Source: CAD feature listing. Evaluate the final solid. Frame: model axes, mm. A direction names the side the tool comes from. Give positions to 0.01 mm unless a question says otherwise; leave off trailing zeros. One line per question, with ' | ' between items. Start each with the question number.
(1) Section A-A, the plane z = 0. State how many separate pieces and enclosed holes the cut face has, plus the area to 3 significant figures.
(2) Ray query, line 1 (X direction, y = 115, z = 17); line 2 (X direction, y = 102, z = 22); line 3 (Z direction, x = -19.5, y = 96). Return the intervals inside material, ascending. Write a range as [from, to].
(3) Access query for faces 1 (the cylindrical face through (-6.93, 62.64, -31.22)), 2 (the cylindrical face through (-1.384, 3.909, 40.762)). Directions: +Z, -Z, +X, -X, +Y, -Y. A direction counts if a zero-diameter tool reaches every point of the face in a straight line with its end or side. Return the directions, or none.
(4) Pin query (flat end, axial travel): pin 1 (6 mm diameter, centred on x = 15, y = 47, fed in from -Z); pin 2 (12 mm diameter, centred on x = 23, z = 27.5, fed in from -Y); pin 3 (5 mm diameter, centred on x = 6.5, y = 77, fed in from -Z); pin 4 (8 mm diameter, centred on x = -33, z = -19.05, fed in from +Y). Return the tip coordinate at first contact, or that it passes through.
Autodesk Inventor part; units mm, degrees
ref_plane "YZ Plane" through (0, 0, 0) normal (1, 0, 0) x (0, 1, 0)
ref_plane "XZ Plane" through (0, 0, 0) normal (0, 1, 0) x (-1, 0, 0)
ref_plane "XY Plane" through (0, 0, 0) normal (0, 0, 1) x (1, 0, 0)
sketch "Sketch1" plane through (0, 0, 0) normal (0, 0, 1) x (1, 0, 0)
  line L0 (0, 0) -> (0, 25.4) construction
  line L1 (30.48, 0) -> (30.48, 127)
  line L2 (0, 0) -> (30.48, 0)
  arc A0 (30.48, 0) -> (30.48, 127) centre (13.335, 63.5) ccw
  line L3 (31.98, 125.0101) -> (31.98, 1.9899)
  arc A1 (31.98, 1.9899) -> (31.98, 125.0101) centre (13.335, 63.5) ccw
  dimension "d0" = 25.4
  dimension "d1" = 30.48
  dimension "d2" = 127
  dimension "d8" = 17.145
  dimension "d9" = 1.5
revolve "Revolution1" add sketch "Sketch1" angle 360 about axis through (0, 0, 0) along (0, 1, 0)
sketch "Sketch2" plane through (0, 0, 0) normal (0, 1, 0) x (-1, 0, 0)
  circle A0 centre (0, 38.1) radius 3
  line L0 (0, 0) -> (0, 38.1) construction
  dimension "d11" = 6
  dimension "d12" = 38.1
extrude "Extrusion1" cut sketch "Sketch2" along normal blind 127
pattern_circular "Circular Pattern1" count 3 over 360 about axis through (0, 63.5, 0) along (0, 1, 0) of "Extrusion1"
properties part number "Buoy 5 HalfSphere"
Check sheet entries:
1) separate pieces: 2 | enclosed holes: 2 | area: 879 mm²
2) line 1: [-51.52, -48.92], [-27.09, -25.3], [25.3, 27.09], [48.92, 51.52] | line 2: [-62.93, -60.95], [-23.21, -21.1], [21.1, 23.21], [60.95, 62.93] | line 3: [-67.77, -65.96], [-25.35, -23.43], [23.43, 25.35], [65.96, 67.77]
3) face 1: none | face 2: +Y, -Y
4) pin 1: z = -76.45 | pin 2: y = 0 | pin 3: z = -77.95 | pin 4: y = 125.91
